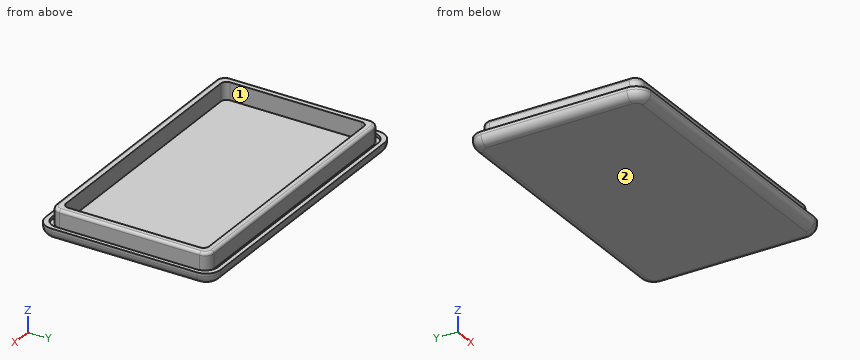
```python
from build123d import *

# Parameters (mm, degrees)
SKETCH_W        = 100
SKETCH_H        = 60
PAD_DEPTH       = 4
FILLET_R        = 5
FILLET001_R     = 3
POCKET001_DEPTH = 1
PAD001_DEPTH    = 5
POCKET_DEPTH    = 6
FILLET002_R     = 1


with BuildPart() as part:
    # Sketch → Pad (new body)
    with BuildSketch(Plane.XY):
        with Locations((50, 30)):
            Rectangle(SKETCH_W, SKETCH_H)
    extrude(amount=PAD_DEPTH)

    # Fillet
    fillet_edges = [part.edges().sort_by_distance(p)[0] for p in [
        (100, 0, 2),
        (0, 0, 2),
        (100, 60, 2),
        (0, 60, 2),
    ]]
    fillet(fillet_edges, radius=FILLET_R)

    # Fillet001
    fillet001_edges = [part.edges().sort_by_distance(p)[0] for p in [
        (50, 60, 0),
    ]]
    fillet(fillet001_edges, radius=FILLET001_R)

    # Sketch008 (on Face6 of Pad) → Pocket001 (cut)
    with BuildSketch(Plane.XY.offset(4)):
        with BuildLine():
            Line((6, 1.5), (94, 1.5))
            ThreePointArc((94, 1.5), (97.181981, 2.818019), (98.5, 6))
            Line((98.5, 6), (98.5, 54))
            ThreePointArc((98.5, 54), (97.181981, 57.181981), (94, 58.5))
            Line((94, 58.5), (6, 58.5))
            ThreePointArc((6, 58.5), (2.818019, 57.181981), (1.5, 54))
            Line((1.5, 54), (1.5, 6))
            ThreePointArc((1.5, 6), (2.818019, 2.818019), (6, 1.5))
        make_face()
        with BuildLine():
            Line((6, 3), (94, 3))
            ThreePointArc((94, 3), (96.12132, 3.87868), (97, 6))
            Line((97, 6), (97, 54))
            ThreePointArc((97, 54), (96.12132, 56.12132), (94, 57))
            Line((94, 57), (6, 57))
            ThreePointArc((6, 57), (3.87868, 56.12132), (3, 54))
            Line((3, 54), (3, 6))
            ThreePointArc((3, 6), (3.87868, 3.87868), (6, 3))
        make_face(mode=Mode.SUBTRACT)
    extrude(amount=-POCKET001_DEPTH, mode=Mode.SUBTRACT)

    # Sketch001 (on Face6 of Pad) → Pad001 (join)
    with BuildSketch(Plane.XY.offset(4)):
        with BuildLine():
            Line((6, 3), (94, 3))
            ThreePointArc((94, 3), (96.12132, 3.87868), (97, 6))
            Line((97, 6), (97, 54))
            ThreePointArc((97, 54), (96.12132, 56.12132), (94, 57))
            Line((94, 57), (6, 57))
            ThreePointArc((6, 57), (3.87868, 56.12132), (3, 54))
            Line((3, 54), (3, 6))
            ThreePointArc((3, 6), (3.87868, 3.87868), (6, 3))
        make_face()
    extrude(amount=PAD001_DEPTH)

    # Sketch009 (on Face44 of Pad001) → Pocket (cut)
    with BuildSketch(Plane.XY.offset(9)):
        with BuildLine():
            Line((7.5, 5.5), (92.5, 5.5))
            ThreePointArc((92.5, 5.5), (93.914214, 6.085786), (94.5, 7.5))
            Line((94.5, 7.5), (94.5, 52.5))
            ThreePointArc((94.5, 52.5), (93.914214, 53.914214), (92.5, 54.5))
            Line((92.5, 54.5), (7.5, 54.5))
            ThreePointArc((7.5, 54.5), (6.085786, 53.914214), (5.5, 52.5))
            Line((5.5, 52.5), (5.5, 7.5))
            ThreePointArc((5.5, 7.5), (6.085786, 6.085786), (7.5, 5.5))
        make_face()
    extrude(amount=-POCKET_DEPTH, mode=Mode.SUBTRACT)

    # Fillet002
    fillet002_edges = [part.edges().sort_by_distance(p)[0] for p in [
        (50, 3, 9),
    ]]
    fillet(fillet002_edges, radius=FILLET002_R)


solid = part.part
```
Read the model definition and answer for the solid it produces. Units are mm, in the model's axes. Face numbers are marked on the shaded views. Give positions to 0.01 mm unless a question says otherwise; leave off trailing zeros. Write each loop counter-clockwise with the first axis right and the second up, starting at its lowest first coordinate (ties: lowest second). Pieces come first, ordered by that corner, then holes. Notation, with made-up numbers: M 0.25,82 L 59.25,82 A20 ccw 59.25,121 Z; hole C 39,27.5 d10. An arc over 180 degrees is marked long. Put each result on its own line as item: value. Start each with the question number.
1. The part is cut by section C-C, the plane y = 9. Give the vertices of the cut face in (x, z), and give its area (3 significant figures).
2. The part is cut by section A-A, the plane z = 6. Give the vertices of the cut face in (x, y).
3. Consider line 1 along X through (y, z) = (19.5, 5.5); line 2 along Y through (x, z) = (77, 4.25); line 3 along X through (y, z) = (6, 3.75). Determine where each line is inside the solid, lowest interval first.
4. The part is cut by section B-B, the plane x = 34. Give the vertices of the cut face in (y, z).
5. For a pull along X with two mould halves and no side action, classify the marked faces 1 and 2 as released by +X, released by -X, zero draft, split by the parting line, or undercut.
6. Each of these flat-tipped pins is pushed along its axis until it touches: pin 1 Ø4 at (x, y) = (34.5, 11.5) entering from +Z; pin 2 Ø1.5 at (x, z) = (34, 6) entering from +Y; pin 3 Ø1.8 at (x, z) = (40, 7) entering from -Y. Where does it stop, or does it pass through?
Final values:
1. outline: M 0,3 A3 ccw 3,0 L 97,0 A3 ccw 100,3 L 100,4 L 98.5,4 L 98.5,3 L 97,3 L 97,8 A1 ccw 96,9 L 94.5,9 L 94.5,3 L 5.5,3 L 5.5,9 L 4,9 A1 ccw 3,8 L 3,3 L 1.5,3 L 1.5,4 L 0,4 Z
1. area: 329 mm²
2. outline: M 3,6 A3 ccw 6,3 L 94,3 A3 ccw 97,6 L 97,54 A3 ccw 94,57 L 6,57 A3 ccw 3,54 Z; hole M 5.5,7.5 A2 ccw 7.5,5.5 L 92.5,5.5 A2 ccw 94.5,7.5 L 94.5,52.5 A2 ccw 92.5,54.5 L 7.5,54.5 A2 ccw 5.5,52.5 Z
3. line 1: x = 3 to 5.5, 94.5 to 97
3. line 2: y = 3 to 5.5, 54.5 to 57
3. line 3: x = 0 to 1.5, 3 to 6.18, 93.82 to 97, 98.5 to 100
4. outline: M 0,3 A3 ccw 3,0 L 57,0 A3 ccw 60,3 L 60,4 L 58.5,4 L 58.5,3 L 57,3 L 57,8 A1 ccw 56,9 L 54.5,9 L 54.5,3 L 5.5,3 L 5.5,9 L 4,9 A1 ccw 3,8 L 3,3 L 1.5,3 L 1.5,4 L 0,4 Z
5. face 1: undercut
5. face 2: zero draft
6. pin 1: stops at z = 3
6. pin 2: stops at y = 57
6. pin 3: stops at y = 3
